Could you check a few things on this model? Use its own coordinates, in mm. Give positions to 0.01 mm unless a question says otherwise; leave off trailing zeros. Loops run counter-clockwise (first coordinate to the right, second up) from the corner with the lowest first, then second, coordinate; pieces in that order, holes last. Notation, with made-up numbers: (3, -33) -> (8, -33) arc R25 cw to (8, -13) -> close; hole circle Ø2 at (70, 59.25). An arc over 180 degrees is marked (long way). Put each result on its own line as item: value.
Autodesk Inventor part; units mm, degrees
ref_plane "YZ Plane" through (0, 0, 0) normal (1, 0, 0) x (0, 1, 0)
ref_plane "XZ Plane" through (0, 0, 0) normal (0, 1, 0) x (-1, 0, 0)
ref_plane "XY Plane" through (0, 0, 0) normal (0, 0, 1) x (1, 0, 0)
sketch "Sketch1" plane through (0, 0, 0) normal (0, 0, 1) x (1, 0, 0)
  arc A0 (-154.1048, 152.1451) -> (-166.8784, 78.2408) centre (-96.4886, 104.1307) ccw construction
  arc A1 (-157.9458, 155.346) -> (-171.571, 76.5148) centre (-96.4886, 104.1307) ccw
  arc A2 (-150.2637, 148.9441) -> (-162.1857, 79.9668) centre (-96.4886, 104.1307) ccw
  arc A3 (-150.2637, 148.9441) -> (-157.9458, 155.346) centre (-154.1048, 152.1451) ccw
  arc A4 (-171.571, 76.5148) -> (-162.1857, 79.9668) centre (-166.8784, 78.2408) ccw
  line L0 (-154.1048, 152.1451) -> (-96.4886, 104.1307) construction
  line L1 (-96.4886, 104.1307) -> (-166.8784, 78.2408) construction
  point P0 (0, 0)
  dimension "d1" = 75
  dimension "d2" = 10
  dimension "d5" = 60
extrude "Extrusion1" add sketch "Sketch1" along normal blind 10
sketch "Sketch2" plane through (0, 0, 10) normal (0, 0, 1) x (1, 0, 0)
  arc A0 (-157.9458, 155.346) -> (-171.571, 76.5148) centre (-96.4886, 104.1307) ccw
  arc A1 (-171.571, 76.5148) -> (-162.1857, 79.9668) centre (-166.8784, 78.2408) ccw
  arc A2 (-150.2637, 148.9441) -> (-162.1857, 79.9668) centre (-96.4886, 104.1307) ccw
  arc A3 (-150.2637, 148.9441) -> (-157.9458, 155.346) centre (-154.1048, 152.1451) ccw
  point P0 (0, 0)
hole "Hole1" at (-154.1048, 152.1451, 10) at (-166.8784, 78.2408, 10) direction (0, 0, -1) diameter 5 end through all
properties part number "ledeplate"
1. I need wall thicknesses on line 1 (Y direction, x = -150.25, z = 2); line 2 (X direction, y = 151.5, z = 7.5); line 3 (Y direction, x = -166.75, z = 1.25). Which ranges of each line are inside material? Lowest first, please.
Recorded:
line 1: y = 148.96 to 155.33
line 2: x = -160.96 to -156.52, -151.69 to -149.15
line 3: y = 73.24 to 75.74, 80.74 to 142.38
2. If we section it at A-A (x = -153): List the corners of the cut face in (y, z) for me, then the cut area to 3 significant figures.
Recorded:
outline: (145.44, 0) -> (149.9, 0) -> (149.9, 10) -> (145.44, 10) -> close; (154.39, 0) -> (157.02, 0) -> (157.02, 10) -> (154.39, 10) -> close
area: 71.0 mm^2
3. If we section it at B-B (z = 8): List the corners of the cut face in (x, y) for me, then the cut area to 3 significant figures.
Recorded:
outline: (-171.57, 76.51) arc R5 ccw to (-162.19, 79.97) arc R70 cw to (-150.26, 148.94) arc R5 ccw to (-157.95, 155.35) arc R80 ccw to start; hole circle Ø5 at (-166.88, 78.24); hole circle Ø5 at (-154.1, 152.15)
area: 825 mm^2
4. If we section it at C-C (y = 126): List the corners of the cut face in (x, z) for me, then the cut area to 3 significant figures.
Recorded:
outline: (-173.44, 0) -> (-162.98, 0) -> (-162.98, 10) -> (-173.44, 10) -> close
area: 105 mm^2
5. Thinking about a two-plate mould opening in Y: for faces 1 (the face through (-175.418, 117.178, 4.93)), 2 (the face through (-168.99, 76.9, 4.93)), 3 (the face through (-167, 118, 0)), which applies, pulls with the +Y half, pulls with the -Y half, needs draft (parallel to the pull), parting line crosses it, or undercut?
Recorded:
face 1: parting line crosses it
face 2: undercut
face 3: needs draft
6. I'm going to push flat-ended pins straight in: pin 1 (4 mm diameter, centred on y = 98, z = 7, fed in from +X); pin 2 (2 mm diameter, centred on y = 108.5, z = 6, fed in from +X); pin 3 (6 mm diameter, centred on x = -158.5, y = 140, fed in from -Z); pin 4 (5 mm diameter, centred on y = 127.5, z = 2.5, fed in from +X). Where does each tip first touch, or does it pass through?
Recorded:
pin 1: stops at x = -166.01
pin 2: stops at x = -166.28
pin 3: stops at z = 0
pin 4: stops at x = -161.53
7. If we section it at D-D (x = -174): List the corners of the cut face in (y, z) for me, then the cut area to 3 significant figures.
Recorded:
outline: (84.33, 0) -> (123.93, 0) -> (123.93, 10) -> (84.33, 10) -> close
area: 396 mm^2
